```python
from build123d import *

# Parameters (mm, degrees)
SKETCH1_R           = 3.75
BOSS_EXTRUDE1_DEPTH = 3
SKETCH5_W           = 8.5
SKETCH5_H           = 8.5
BOSS_EXTRUDE3_DEPTH = 5
CUT_EXTRUDE4_DEPTH  = 30
SKETCH2_W           = 10
SKETCH2_H           = 37.69615365
SKETCH2_W_2         = 37.69615365
SKETCH2_H_2         = 10
BOSS_EXTRUDE4_DEPTH = 1.5
FILLET1_R           = 5
FILLET2_R           = 6


with BuildPart() as part:
    # Sketch1 → Boss-Extrude1 (new body)
    with BuildSketch(Plane(origin=(0, 0, 0), x_dir=(1, 0, 0), z_dir=(0, 1, 0))):
        with Locations(Location((0, 0, 0), (0, 0, 270))):
            Circle(SKETCH1_R)
    extrude(amount=BOSS_EXTRUDE1_DEPTH)

    # Sketch5 → Boss-Extrude3 (add)
    with BuildSketch(Plane(origin=(0, 3, 0), x_dir=(1, 0, 0), z_dir=(0, 1, 0))):
        Rectangle(SKETCH5_W, SKETCH5_H)
    extrude(amount=BOSS_EXTRUDE3_DEPTH)

    # Sketch19 → Cut-Extrude4 (cut)
    with BuildSketch(Plane.ZY.offset(4.25)):
        Polygon((-4.25, 8), (4.25, 8), (4.25, 5.722431864), align=None)
    extrude(amount=-CUT_EXTRUDE4_DEPTH, mode=Mode.SUBTRACT)

    # Sketch2 → Boss-Extrude4 (add)
    with BuildSketch(Plane.XZ):
        Rectangle(SKETCH2_W, SKETCH2_H)
        Rectangle(SKETCH2_W_2, SKETCH2_H_2)
    extrude(amount=BOSS_EXTRUDE4_DEPTH)

    # Fillet1
    fillet1_edges = [part.edges().sort_by_distance(p)[0] for p in [
        (18.848076825, -0.75, -5),
        (5, -0.75, -18.848076825),
        (-5, -0.75, -18.848076825),
        (-18.848076825, -0.75, -5),
        (-18.848076825, -0.75, 5),
        (18.848076825, -0.75, 5),
        (5, -0.75, 18.848076825),
        (-5, -0.75, 18.848076825),
    ]]
    fillet(fillet1_edges, radius=FILLET1_R - 0.0001)  # a hair under: the kernel refuses the full size

    # Fillet2
    fillet2_edges = [part.edges().sort_by_distance(p)[0] for p in [
        (5, -0.75, -5),
        (-5, -0.75, 5),
        (-5, -0.75, -5),
        (5, -0.75, 5),
    ]]
    fillet(fillet2_edges, radius=FILLET2_R)


solid = part.part
```
Input: part model. Units: mm. Frame: model coordinates. A direction names the side the tool comes from. Coordinates: 2 decimals unless noted, no trailing zeros. Order: outer loops, then holes, each group sorted by start corner. A loop starts at its lowest first (then second) coordinate and runs counter-clockwise, first axis right, second up. Notation, with made-up numbers: (6.25, -14.5) - (23.25, -14.5) arc R21 ccw to (23.25, 8.5) - close; hole circle Ø2 at (-37, -22). An arc over 180 degrees is marked (long way). Return JSON: item names as keys, results as strings.
Q1. Cut plane A-A (y = 1.25). Return loops of the section in (x, z).
The answers:
{"outline": "circle Ø7.5 at (0, 0)"}
Q2. Cut plane D-D (z = -1). Return loops of the section in (x, y), then the cut area to 3 significant figures.
The answers:
{"outline": "(-18.75, -1.5) - (18.75, -1.5) - (18.75, 0) - (3.61, 0) - (3.61, 3) - (4.25, 3) - (4.25, 7.13) - (-4.25, 7.13) - (-4.25, 3) - (-3.61, 3) - (-3.61, 0) - (-18.75, 0) - close", "area": "113 mm2"}
Q3. Cut plane C-C (x = -9.5). Return loops of the section in (y, z).
The answers:
{"outline": "(-1.5, -5.19) - (0, -5.19) - (0, 5.19) - (-1.5, 5.19) - close"}
Q4. Cut plane B-B (z = -12). Return loops of the section in (x, y), then the cut area to 3 significant figures.
The answers:
{"outline": "(-5, -1.5) - (5, -1.5) - (5, 0) - (-5, 0) - close", "area": "15.0 mm2"}
Q5. Access query for faces 1 (the flat face through (4.25, 5, 0)), 2 (the flat face through (-12, -1, 5)), 3 (the flat face through (5, -1, 12)). Directions: +Z, -Z, +X, -X, +Y, -Y. A direction counts if a zero-diameter tool reaches every point of the face in a straight line with its end or side. Return the directions, or none.
The answers:
{"face 1": "+Z, -Z, +X, +Y", "face 2": "+Z, -X, +Y, -Y", "face 3": "+Z, +X, +Y, -Y"}
Q6. Draft query along Y for faces 4 (the flat face through (-4.25, 5, 0)), 5 (the flat face through (-4, 3, 0)), 6 (the flat face through (-0.059, 6.845, 0.059)), 7 (the flat face through (0, -1.5, 0)). Return one class per face: +Y half, -Y half, draft (parallel to the pull), parting line (faces both ways), or undercut.
The answers:
{"face 4": "draft", "face 5": "undercut", "face 6": "+Y half", "face 7": "-Y half"}
Q7. First-contact query: pin 1 (4 mm diameter, centred on x = 0, y = 6, fed in from -Z); pin 2 (0.8 mm diameter, centred on x = -13, y = -1, fed in from -Z); pin 3 (0.8 mm diameter, centred on x = -12, y = -1, fed in from +Z). Flat tips, straight axial feed; report the tip coordinate or a pass-through.
The answers:
{"pin 1": "stops at z = -4.25", "pin 2": "stops at z = -5", "pin 3": "stops at z = 5"}
Q8. Ray query, probe 1 along Z at (x, y) = (-13, -0.5); probe 2 along X at (y, z) = (-0.75, 16.5); probe 3 along Y at (x, z) = (-17, 3). Return the intervals inside material, ascending.
The answers:
{"probe 1": "z = -5 to 5", "probe 2": "x = -4.24 to 4.24", "probe 3": "y = -1.5 to 0"}
